Read the model definition and answer for the solid it produces. Units are mm, in the model's axes. Face numbers are marked on the shaded views. A direction names the side the tool comes from. Give positions to 0.01 mm unless a question says otherwise; leave off trailing zeros. Order: outer loops, then holes, each group sorted by start corner. A loop starts at its lowest first (then second) coordinate and runs counter-clockwise, first axis right, second up. Notation, with made-up numbers: (31.25, -34) - (39.25, -34) arc R20 cw to (39.25, -19) - close; hole circle Ø8 at (20.5, 42.25). An arc over 180 degrees is marked (long way). One line per item, written item: value. Start each with the question number.
```python
from build123d import *

# Parameters (mm, degrees)
CYLINDER383_R             = 1.25
CYLINDER383_DEPTH         = 10
CYLINDER384_R             = 1.25
CYLINDER384_DEPTH         = 10
CYLINDER385_R             = 1.25
CYLINDER385_DEPTH         = 10
CYLINDER386_R             = 1.25
CYLINDER386_DEPTH         = 10
CYLINDER388_R             = 1.25
CYLINDER388_DEPTH         = 10
CYLINDER387_R             = 1.25
CYLINDER387_DEPTH         = 10
CYLINDER381_R             = 1.25
CYLINDER381_DEPTH         = 10
CYLINDER382_R             = 1.25
CYLINDER382_DEPTH         = 10
BOX267_W                  = 10
BOX267_H                  = 10
BOX267_DEPTH              = 10
CYLINDER377_R             = 1.6
CYLINDER377_DEPTH         = 10
CYLINDER378_R             = 1.6
CYLINDER378_DEPTH         = 10
FUSION322_PLACEMENT_ANGLE = 120
CYLINDER380_R             = 1.6
CYLINDER380_DEPTH         = 10
CYLINDER379_R             = 1.6
CYLINDER379_DEPTH         = 10
CYLINDER375_R             = 1.6
CYLINDER375_DEPTH         = 10
CYLINDER376_R             = 1.6
CYLINDER376_DEPTH         = 10
FUSION321_PLACEMENT_ANGLE = 60
FUSION324_PLACEMENT_ANGLE = 30
CUT276_PLACEMENT_ANGLE    = 90
CYLINDER374_R             = 18.7
CYLINDER374_DEPTH         = 75
CYLINDER373_R             = 7
CYLINDER373_DEPTH         = 10
CYLINDER372_R             = 20.5
CYLINDER372_DEPTH         = 34
BOX266_W                  = 34
BOX266_H                  = 80
BOX266_DEPTH              = 17
CHAMFER026_SIZE           = 8
FILLET103_R               = 2


with BuildPart() as cylinder383:
    # Cylinder383 → Cylinder383 (new body)
    with BuildSketch(Plane(origin=(87.5, 71, 14), x_dir=(1, 0, 0), z_dir=(0, -1, 0))):
        Circle(CYLINDER383_R)
    extrude(amount=CYLINDER383_DEPTH)


with BuildPart() as cylinder384:
    # Cylinder384 → Cylinder384 (new body)
    with BuildSketch(Plane(origin=(87.5, 1, 14), x_dir=(1, 0, 0), z_dir=(0, -1, 0))):
        Circle(CYLINDER384_R)
    extrude(amount=CYLINDER384_DEPTH)


with BuildPart() as fusion332:
    # Fusion332 base: copy of Cylinder384
    add(cylinder384.part)

    # Fusion332: union Cylinder383
    add(cylinder383.part)


with BuildPart() as fusion332_1:
    # Fusion332 placement: moved
    add(fusion332.part.moved(Location((251.5, 0, 0))))


with BuildPart() as cylinder385:
    # Cylinder385 → Cylinder385 (new body)
    with BuildSketch(Plane(origin=(87.5, 71, 14), x_dir=(1, 0, 0), z_dir=(0, -1, 0))):
        Circle(CYLINDER385_R)
    extrude(amount=CYLINDER385_DEPTH)


with BuildPart() as cylinder386:
    # Cylinder386 → Cylinder386 (new body)
    with BuildSketch(Plane(origin=(87.5, 1, 14), x_dir=(1, 0, 0), z_dir=(0, -1, 0))):
        Circle(CYLINDER386_R)
    extrude(amount=CYLINDER386_DEPTH)


with BuildPart() as fusion333:
    # Fusion333 base: copy of Cylinder386
    add(cylinder386.part)

    # Fusion333: union Cylinder385
    add(cylinder385.part)


with BuildPart() as fusion333_1:
    # Fusion333 placement: moved
    add(fusion333.part.moved(Location((261.5, 0, 0))))


with BuildPart() as cylinder388:
    # Cylinder388 → Cylinder388 (new body)
    with BuildSketch(Plane(origin=(87.5, 71, 14), x_dir=(1, 0, 0), z_dir=(0, -1, 0))):
        Circle(CYLINDER388_R)
    extrude(amount=CYLINDER388_DEPTH)


with BuildPart() as cylinder387:
    # Cylinder387 → Cylinder387 (new body)
    with BuildSketch(Plane(origin=(87.5, 1, 14), x_dir=(1, 0, 0), z_dir=(0, -1, 0))):
        Circle(CYLINDER387_R)
    extrude(amount=CYLINDER387_DEPTH)


with BuildPart() as fusion331:
    # Fusion331 base: copy of Cylinder387
    add(cylinder387.part)

    # Fusion331: union Cylinder388
    add(cylinder388.part)


with BuildPart() as fusion331_1:
    # Fusion331 placement: moved
    add(fusion331.part.moved(Location((270.5, 0, 0))))


with BuildPart() as cylinder381:
    # Cylinder381 → Cylinder381 (new body)
    with BuildSketch(Plane(origin=(87.5, 71, 14), x_dir=(1, 0, 0), z_dir=(0, -1, 0))):
        Circle(CYLINDER381_R)
    extrude(amount=CYLINDER381_DEPTH)


with BuildPart() as cylinder382:
    # Cylinder382 → Cylinder382 (new body)
    with BuildSketch(Plane(origin=(87.5, 1, 14), x_dir=(1, 0, 0), z_dir=(0, -1, 0))):
        Circle(CYLINDER382_R)
    extrude(amount=CYLINDER382_DEPTH)


with BuildPart() as fusion330:
    # Fusion334 base: copy of Cylinder382
    add(cylinder382.part)

    # Fusion334: union Cylinder381
    add(cylinder381.part)


with BuildPart() as fusion330_1:
    # Fusion334 placement: moved
    add(fusion330.part.moved(Location((242.5, 0, 0))))

    # Fusion330: union Fusion332, Fusion333, Fusion331
    add(fusion332_1.part)
    add(fusion333_1.part)
    add(fusion331_1.part)


with BuildPart() as fusion330_2:
    # Fusion330 placement: moved
    add(fusion330_1.part.moved(Location((0, 0, -8))))


with BuildPart() as fusion326:
    # Fusion326 base: copy of Cylinder384
    add(cylinder384.part)

    # Fusion326: union Cylinder383
    add(cylinder383.part)


with BuildPart() as fusion326_1:
    # Fusion326 placement: moved
    add(fusion326.part.moved(Location((251.5, 0, 0))))


with BuildPart() as fusion327:
    # Fusion327 base: copy of Cylinder386
    add(cylinder386.part)

    # Fusion327: union Cylinder385
    add(cylinder385.part)


with BuildPart() as fusion327_1:
    # Fusion327 placement: moved
    add(fusion327.part.moved(Location((261.5, 0, 0))))


with BuildPart() as fusion328:
    # Fusion328 base: copy of Cylinder387
    add(cylinder387.part)

    # Fusion328: union Cylinder388
    add(cylinder388.part)


with BuildPart() as fusion328_1:
    # Fusion328 placement: moved
    add(fusion328.part.moved(Location((270.5, 0, 0))))


with BuildPart() as fusion335:
    # Fusion325 base: copy of Cylinder382
    add(cylinder382.part)

    # Fusion325: union Cylinder381
    add(cylinder381.part)


with BuildPart() as fusion335_1:
    # Fusion325 placement: moved
    add(fusion335.part.moved(Location((242.5, 0, 0))))

    # Fusion329: union Fusion326, Fusion327, Fusion328
    add(fusion326_1.part)
    add(fusion327_1.part)
    add(fusion328_1.part)

    # Fusion335: union Fusion330
    add(fusion330_2.part)


with BuildPart() as cube347:
    # Box267 → Box267 (new body)
    with BuildSketch(Plane.XY):
        with Locations((5, 5)):
            Rectangle(BOX267_W, BOX267_H)
    extrude(amount=BOX267_DEPTH)


with BuildPart() as cylinder377:
    # Cylinder377 → Cylinder377 (new body)
    with BuildSketch(Plane(origin=(15.5, 0, 0), x_dir=(1, 0, 0), z_dir=(0, 0, 1))):
        Circle(CYLINDER377_R)
    extrude(amount=CYLINDER377_DEPTH)


with BuildPart() as fusion322:
    # Cylinder378 → Cylinder378 (new body)
    with BuildSketch(Plane(origin=(-15.5, 0, 0), x_dir=(1, 0, 0), z_dir=(0, 0, 1))):
        Circle(CYLINDER378_R)
    extrude(amount=CYLINDER378_DEPTH)

    # Fusion322: union Cylinder377
    add(cylinder377.part)


with BuildPart() as fusion322_1:
    # Fusion322 placement: moved
    add(fusion322.part.rotate(Axis((0, 0, 0), (0, 0, 1)), FUSION322_PLACEMENT_ANGLE))


with BuildPart() as cylinder380:
    # Cylinder380 → Cylinder380 (new body)
    with BuildSketch(Plane(origin=(15.5, 0, 0), x_dir=(1, 0, 0), z_dir=(0, 0, 1))):
        Circle(CYLINDER380_R)
    extrude(amount=CYLINDER380_DEPTH)


with BuildPart() as fusion323:
    # Cylinder379 → Cylinder379 (new body)
    with BuildSketch(Plane(origin=(-15.5, 0, 0), x_dir=(1, 0, 0), z_dir=(0, 0, 1))):
        Circle(CYLINDER379_R)
    extrude(amount=CYLINDER379_DEPTH)

    # Fusion323: union Cylinder380
    add(cylinder380.part)


with BuildPart() as cylinder375:
    # Cylinder375 → Cylinder375 (new body)
    with BuildSketch(Plane(origin=(15.5, 0, 0), x_dir=(1, 0, 0), z_dir=(0, 0, 1))):
        Circle(CYLINDER375_R)
    extrude(amount=CYLINDER375_DEPTH)


with BuildPart() as holes003:
    # Cylinder376 → Cylinder376 (new body)
    with BuildSketch(Plane(origin=(-15.5, 0, 0), x_dir=(1, 0, 0), z_dir=(0, 0, 1))):
        Circle(CYLINDER376_R)
    extrude(amount=CYLINDER376_DEPTH)

    # Fusion321: union Cylinder375
    add(cylinder375.part)


with BuildPart() as holes003_1:
    # Fusion321 placement: moved
    add(holes003.part.rotate(Axis((0, 0, 0), (0, 0, 1)), FUSION321_PLACEMENT_ANGLE))

    # Fusion324: union Fusion322, Fusion323
    add(fusion322_1.part)
    add(fusion323.part)


with BuildPart() as holes003_2:
    # Fusion324 placement: moved
    add(holes003_1.part.rotate(Axis((0, 0, 0), (0, 0, 1)), FUSION324_PLACEMENT_ANGLE))

    # Cut276: cut Cube347
    add(cube347.part, mode=Mode.SUBTRACT)


with BuildPart() as holes003_3:
    # Cut276 placement: moved
    add(holes003_2.part.moved(Location((327, 31, 5))).rotate(Axis((327, 31, 5), (0, 1, 0)), CUT276_PLACEMENT_ANGLE))


with BuildPart() as cylinder374:
    # Cylinder374 → Cylinder374 (new body)
    with BuildSketch(Plane(origin=(336, 31, 5), x_dir=(0, 0, -1), z_dir=(1, 0, 0))):
        Circle(CYLINDER374_R)
    extrude(amount=CYLINDER374_DEPTH)


with BuildPart() as cylinder373:
    # Cylinder373 → Cylinder373 (new body)
    with BuildSketch(Plane(origin=(327, 31, 12), x_dir=(0, 0, -1), z_dir=(1, 0, 0))):
        Circle(CYLINDER373_R)
    extrude(amount=CYLINDER373_DEPTH)


with BuildPart() as cylinder372:
    # Cylinder372 → Cylinder372 (new body)
    with BuildSketch(Plane(origin=(326, 31, 4.5), x_dir=(0, 0, -1), z_dir=(1, 0, 0))):
        Circle(CYLINDER372_R)
    extrude(amount=CYLINDER372_DEPTH)


with BuildPart() as motor_support_wide:
    # Box266 → Box266 (new body)
    with BuildSketch(Plane(origin=(326, -9, 1.5), x_dir=(1, 0, 0), z_dir=(0, 0, 1))):
        with Locations((17, 40)):
            Rectangle(BOX266_W, BOX266_H)
    extrude(amount=BOX266_DEPTH)

    # Fusion336: union Cylinder372
    add(cylinder372.part)

    # Chamfer026
    chamfer026_edges = [motor_support_wide.edges().sort_by_distance(p)[0] for p in [
        (343, 51.2793, 1.5),
        (343, 10.7207, 1.5),
    ]]
    chamfer(chamfer026_edges, length=CHAMFER026_SIZE)

    # Fillet103
    fillet103_edges = [motor_support_wide.edges().sort_by_distance(p)[0] for p in [
        (343, 71, 1.5),
        (343, 71, 18.5),
        (343, -9, 18.5),
        (343, -9, 1.5),
    ]]
    fillet(fillet103_edges, radius=FILLET103_R)


with BuildPart() as motor_support_wide_1:
    # Fillet103 placement: moved
    add(motor_support_wide.part.moved(Location((1, 0, 0))))

    # Cut277: cut Cylinder373
    add(cylinder373.part, mode=Mode.SUBTRACT)

    # Cut278: cut Cylinder374
    add(cylinder374.part, mode=Mode.SUBTRACT)

    # Cut279: cut holes003
    add(holes003_3.part, mode=Mode.SUBTRACT)

    # Cut280: cut Fusion335
    add(fusion335_1.part, mode=Mode.SUBTRACT)


with BuildPart() as motor_support_wide_2:
    # Cut280 placement: moved
    add(motor_support_wide_1.part.moved(Location((86, 0, 0))))


solid = motor_support_wide_2.part
```
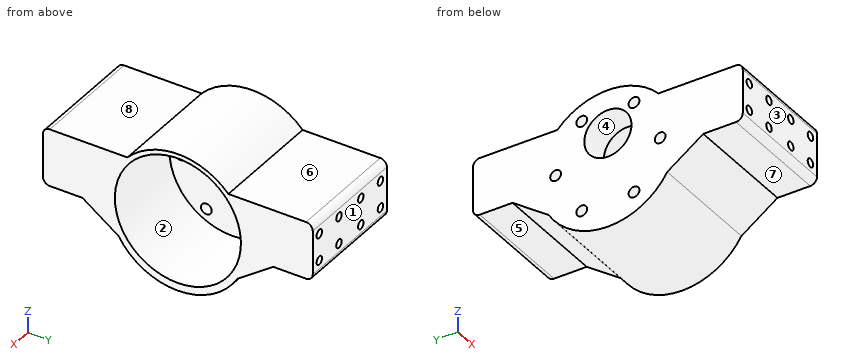
1) Find the intervals of material crossed by probe 1 along Z at (x, y) = (444, -6); probe 2 along Y at (x, z) = (438, 5); probe 3 along Z at (x, y) = (427, 31.5), in increasing order. Write a range as from..to.
2) Each of these flat-tipped pins is pushed along its axis until it touches: pin 1 (3 mm diameter, centred on x = 421, y = 31, fed in from +Z); pin 2 (6 mm diameter, centred on x = 427.5, z = -5, fed in from -Y); pin 3 (1.5 mm diameter, centred on x = 425, z = 14, fed in from +Y). Where does it stop, or does it pass through?
3) Section C-C on z = -8 is taken. Write down the section's boundary in (x, y).
4) Section A-A on y = 66 is taken. Give the number of separate pieces and of enclosed holes in the cut face, plus the area to 3 significant figures.
5) For the marked faces 5, 6, 7 and 8, determine the directions among +Z, -Z, +X, -X, +Y, -Y from which every point of the face is accessible in a straight line to the end or side of a thin tool.
6) The mould has two halves that part along Y. Classify the marked faces 1, 2, 3 and 4: +Y half, -Y half, draft (parallel to the pull), parting line (faces both ways), or undercut.
7) Section B-B on y = 23 is taken. Write down the section's boundary in (x, z).
Solved:
1. probe 1: z = 1.5..4.75, 7.25..12.75, 15.25..18.5
1. probe 2: y = -9..12.3, 49.7..71
1. probe 3: z = -15.99..-13.69, 23.69..24.99
2. pin 1: stops at z = 25
2. pin 2: stops at y = 7.69
2. pin 3: stops at y = 61
3. outline: (413, 14.75) - (447, 14.75) - (447, 17.56) - (422, 17.56) - (422, 21.71) - (413, 21.71) - close; (413, 24.79) - (422, 24.79) - (422, 37.21) - (413, 37.21) - close; (413, 40.29) - (422, 40.29) - (422, 44.44) - (447, 44.44) - (447, 47.25) - (413, 47.25) - close
4. separate pieces: 1
4. enclosed holes: 8
4. area: 539 mm2
5. face 5: -Z, +X, -X, +Y
5. face 6: +Z, +X, -X, +Y
5. face 7: -Z, +X, -X, -Y
5. face 8: +Z, +X, -X, -Y
6. face 1: +Y half
6. face 2: undercut
6. face 3: -Y half
6. face 4: undercut
7. outline: (413, -14.37) - (447, -14.37) - (447, -11.9) - (422, -11.9) - (422, -10) - (413, -10) - close; (413, -6.84) - (422, -6.84) - (422, 16.84) - (413, 16.84) - close; (413, 20) - (422, 20) - (422, 21.9) - (447, 21.9) - (447, 23.37) - (413, 23.37) - close
